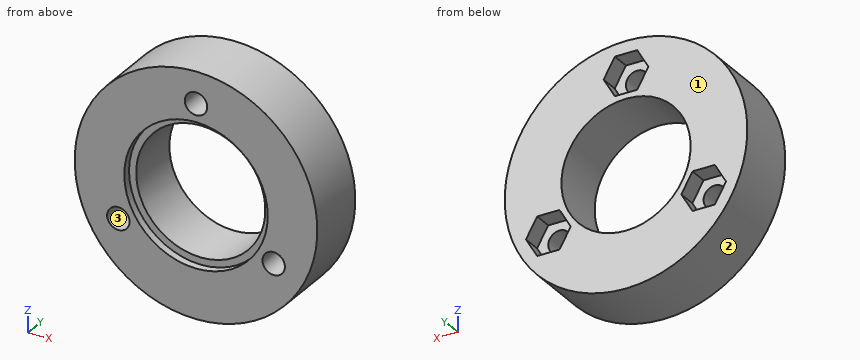
```python
from build123d import *

# Parameters (mm, degrees)
SKETCH1_R           = 23
SKETCH1_R_2         = 12.25
BOSS_EXTRUDE1_DEPTH = 12
SKETCH2_R           = 13.6
CUT_EXTRUDE1_DEPTH  = 1.5
SKETCH3_R           = 2.125
CUT_EXTRUDE2_DEPTH  = 35.669871647
CUT_EXTRUDE3_DEPTH  = 3.5


with BuildPart() as part:
    # Sketch1 → Boss-Extrude1 (new body)
    with BuildSketch(Plane(origin=(0, 0, 0), x_dir=(1, 0, 0), z_dir=(0, 1, 0))):
        with Locations(Location((0, 0, 0), (0, 0, 270))):
            Circle(SKETCH1_R)
        with Locations(Location((0, 0, 0), (0, 0, 270))):
            Circle(SKETCH1_R_2, mode=Mode.SUBTRACT)
    extrude(amount=BOSS_EXTRUDE1_DEPTH)

    # Sketch2 → Cut-Extrude1 (cut)
    with BuildSketch(Plane.XZ):
        with Locations(Location((0, 0, 0), (0, 0, 270))):
            Circle(SKETCH2_R)
    extrude(amount=-CUT_EXTRUDE1_DEPTH, mode=Mode.SUBTRACT)

    # Sketch3 → Cut-Extrude2 (cut, through all)
    with BuildSketch(Plane(origin=(0, 12, 0), x_dir=(1, 0, 0), z_dir=(0, 1, 0))):
        with Locations(Location((0, -17, 0), (0, 0, 270))):
            Circle(SKETCH3_R)
        with Locations(Location((-14.722431864, 8.5, 0), (0, 0, 270))):
            Circle(SKETCH3_R)
        with Locations(Location((14.722431864, 8.5, 0), (0, 0, 270))):
            Circle(SKETCH3_R)
    extrude(amount=-CUT_EXTRUDE2_DEPTH, mode=Mode.SUBTRACT)

    # Sketch4 → Cut-Extrude3 (cut)
    with BuildSketch(Plane(origin=(0, 12, 0), x_dir=(1, 0, 0), z_dir=(0, 1, 0))):
        Polygon((-16.844194104, 4.825), (-12.600669625, 4.825), (-10.478907386, 8.5), (-12.600669625, 12.175), (-16.844194104, 12.175), (-18.965956343, 8.5), align=None)
        Polygon((4.243524479, -17), (2.121762239, -13.325), (-2.121762239, -13.325), (-4.243524479, -17), (-2.121762239, -20.675), (2.121762239, -20.675), align=None)
        Polygon((12.600669625, 12.175), (10.478907386, 8.5), (12.600669625, 4.825), (16.844194104, 4.825), (18.965956343, 8.5), (16.844194104, 12.175), align=None)
    extrude(amount=-CUT_EXTRUDE3_DEPTH, mode=Mode.SUBTRACT)


solid = part.part
```
Design review of the part built by this model. Coordinates are the model's own, in mm. Face numbers are marked on the shaded views. Round coordinates to 2 decimals unless told otherwise and drop trailing zeros. Write each loop counter-clockwise with the first axis right and the second up, starting at its lowest first coordinate (ties: lowest second). Pieces come first, ordered by that corner, then holes. Notation, with made-up numbers: (85, -34) -> (110, -34) arc R20 ccw to (110, -28) -> close; hole circle Ø1 at (67.25, 33). An arc over 180 degrees is marked (long way). Answer in a Markdown table with one row per item.
Q1. Clearance check with flat-ended pins moving along their axes: pin 1 Ø1.8 at (x, y) = (-15, 9.5) entering from -Z; pin 2 Ø6 at (x, z) = (16, -8) entering from +Y; pin 3 Ø1.5 at (y, z) = (5.5, 4.5) entering from -X; pin 4 Ø1 at (x, y) = (-14, 10.5) entering from +Z. State where each tip first meets the part, or that it passes through.
The answers:
| item | result |
|---|---|
| pin 1 | z = -18.17 |
| pin 2 | y = 12 |
| pin 3 | x = -22.69 |
| pin 4 | z = 18.62 |
Q2. Take a section at B-B, the plane z = -2. State the section outline as (x, y) points.
The answers:
| item | result |
|---|---|
| outline | (-22.91, 0) -> (-13.45, 0) -> (-13.45, 1.5) -> (-12.09, 1.5) -> (-12.09, 12) -> (-22.91, 12) -> close; (12.09, 1.5) -> (13.45, 1.5) -> (13.45, 0) -> (22.91, 0) -> (22.91, 12) -> (12.09, 12) -> close |
Q3. To check wall thickness, follow L1, parallel to Z at x = 0.5, y = 2.75; L2, parallel to X at y = 3.75, z = -8.5; L3, parallel to Y at x = 4.5, z = 12.5. State the ranges of each line that lie inside material, in increasing order. Write a range as [from, to].
The answers:
| item | result |
|---|---|
| L1 | [-22.99, -12.24], [12.24, 14.93], [19.07, 22.99] |
| L2 | [-21.37, -16.85], [-12.6, -8.82], [8.82, 12.6], [16.85, 21.37] |
| L3 | [1.5, 12] |
Q4. Draft analysis for pull direction X (two halves, no side actions). For the marked faces 1, 2 and 3, state which applies: +X half, -X half, draft (parallel to the pull), parting line (faces both ways), or undercut.
The answers:
| item | result |
|---|---|
| face 1 | draft |
| face 2 | parting line |
| face 3 | undercut |
Q5. Take a section at C-C, the plane y = 9.25. State the section outline as (x, z) points (3 decimals), then the cut area to 3 significant figures.
The answers:
| item | result |
|---|---|
| outline | circle Ø46 at (0, 0); hole (-18.966, -8.5) -> (-16.844, -12.175) -> (-12.601, -12.175) -> (-10.479, -8.5) -> (-12.601, -4.825) -> (-16.844, -4.825) -> close; hole circle Ø24.5 at (0, 0); hole (-4.244, 17) -> (-2.122, 13.325) -> (2.122, 13.325) -> (4.244, 17) -> (2.122, 20.675) -> (-2.122, 20.675) -> close; hole (10.479, -8.5) -> (12.601, -12.175) -> (16.844, -12.175) -> (18.966, -8.5) -> (16.844, -4.825) -> (12.601, -4.825) -> close |
| area | 1,050 mm² |
Q6. Take a section at A-A, the plane x = 0. State the section outline as (y, z) points (3 decimals).
The answers:
| item | result |
|---|---|
| outline | (0, -23) -> (12, -23) -> (12, -12.25) -> (1.5, -12.25) -> (1.5, -13.6) -> (0, -13.6) -> close; (0, 13.6) -> (1.5, 13.6) -> (1.5, 12.25) -> (12, 12.25) -> (12, 13.325) -> (8.5, 13.325) -> (8.5, 14.875) -> (0, 14.875) -> close; (0, 19.125) -> (8.5, 19.125) -> (8.5, 20.675) -> (12, 20.675) -> (12, 23) -> (0, 23) -> close |
Q7. Take a section at D-D, the plane y = 4.75. State the section outline as (x, z) points (3 decimals), then the cut area to 3 significant figures.
The answers:
| item | result |
|---|---|
| outline | circle Ø46 at (0, 0); hole circle Ø4.25 at (-14.722, -8.5); hole circle Ø24.5 at (0, 0); hole circle Ø4.25 at (0, 17); hole circle Ø4.25 at (14.722, -8.5) |
| area | 1,150 mm² |
